from build123d import *

# Parameters (mm, degrees)
SKETCH1_R                            = 4.7625
BOSS_EXTRUDE1_DEPTH                  = 36.5125
F_10_32_TAPPED_HOLE2_D               = 4.0386
F_10_32_TAPPED_HOLE2_DEPTH           = 12.02944
F_10_32_TAPPED_HOLE2_TIP             = 1.213317848
F_10_32_TAPPED_HOLE2_ON_FACE_2_D     = 4.0386
F_10_32_TAPPED_HOLE2_ON_FACE_2_DEPTH = 12.02944
F_10_32_TAPPED_HOLE2_ON_FACE_2_TIP   = 1.213317848


with BuildPart() as part:
    # Sketch1 → Boss-Extrude1 (new, symmetric)
    with BuildSketch(Plane.XY):
        Circle(SKETCH1_R)
    extrude(amount=BOSS_EXTRUDE1_DEPTH, both=True)

    # #10-32 Tapped Hole2
    with Locations(Plane(origin=(0, 0, -36.5125), x_dir=(-1, 0, 0), z_dir=(0, 0, -1))):
        with Locations((0, 0)):
            Hole(F_10_32_TAPPED_HOLE2_D / 2, depth=F_10_32_TAPPED_HOLE2_DEPTH)
            with Locations((0, 0, -(F_10_32_TAPPED_HOLE2_DEPTH + F_10_32_TAPPED_HOLE2_TIP / 2))):  # 118° drill point
                Cone(0, F_10_32_TAPPED_HOLE2_D / 2, F_10_32_TAPPED_HOLE2_TIP, mode=Mode.SUBTRACT)

    # #10-32 Tapped Hole2 on face 2
    with Locations(Plane.XY.offset(36.5125)):
        with Locations((0, 0)):
            Hole(F_10_32_TAPPED_HOLE2_ON_FACE_2_D / 2, depth=F_10_32_TAPPED_HOLE2_ON_FACE_2_DEPTH)
            with Locations((0, 0, -(F_10_32_TAPPED_HOLE2_ON_FACE_2_DEPTH + F_10_32_TAPPED_HOLE2_ON_FACE_2_TIP / 2))):  # 118° drill point
                Cone(0, F_10_32_TAPPED_HOLE2_ON_FACE_2_D / 2, F_10_32_TAPPED_HOLE2_ON_FACE_2_TIP, mode=Mode.SUBTRACT)


solid = part.part
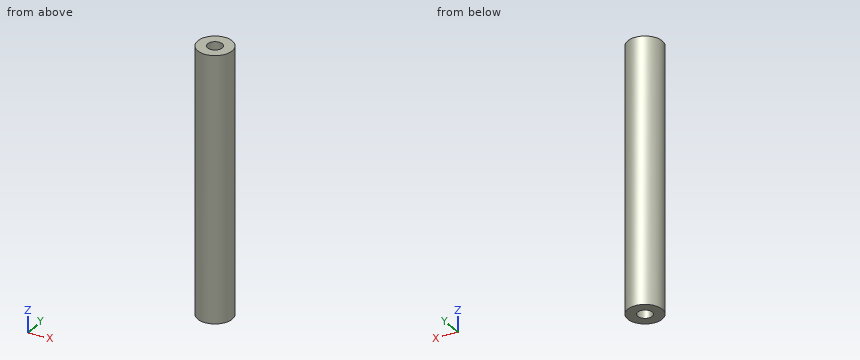
Design review of the part built by this model. Coordinates are the model's own, in mm. Give positions to 0.01 mm unless a question says otherwise; leave off trailing zeros. Loops run counter-clockwise (first coordinate to the right, second up) from the corner with the lowest first, then second, coordinate; pieces in that order, holes last. Notation, with made-up numbers: (-24, -22.75) -> (9, -22.75) arc R21 cw to (9, 9.25) -> close; hole circle Ø6 at (46.25, -35.5). An arc over 180 degrees is marked (long way). One line per question, with ' | ' between items. Start each with the question number.
(1) For line 1 (Y direction, x = 0, z = 32); line 2 (X direction, y = -0.25, z = 16); line 3 (Y direction, x = -3, z = -14), list the stretches that pass through material, from the lowest coordinate up.
(2) We need section C-C (x = -2.75). State the section outline as (y, z) points.
(3) Insertion check: P1, Ø3, axis at x = -3, z = 1.5, coming from the +Y side; P2, Ø2.5, axis at x = 0, y = 0, coming from the -Z side. Each pin has a flat end and moves straight along its axis. Give the tip position at first contact, or say it passes through.
(4) We need section B-B (y = 3). State the section outline as (x, z) points, and give its area (3 significant figures).
(5) We need section A-A (z = 25.5). State the section outline as (x, y) points (1 decimal).
The answers:
1) line 1: y = -4.76 to -2.02, 2.02 to 4.76 | line 2: x = -4.76 to 4.76 | line 3: y = -3.7 to 3.7
2) outline: (-3.89, -36.51) -> (3.89, -36.51) -> (3.89, 36.51) -> (-3.89, 36.51) -> close
3) P1: stops at y = 4.52 | P2: stops at z = -24.02
4) outline: (-3.7, -36.51) -> (3.7, -36.51) -> (3.7, 36.51) -> (-3.7, 36.51) -> close | area: 540 mm^2
5) outline: circle Ø9.5 at (0, 0); hole circle Ø4 at (0, 0)
